Design review of the part built by this model. Coordinates are the model's own, in mm. A direction names the side the tool comes from. Give positions to 0.01 mm unless a question says otherwise; leave off trailing zeros. Write each loop counter-clockwise with the first axis right and the second up, starting at its lowest first coordinate (ties: lowest second). Pieces come first, ordered by that corner, then holes.
```python
from build123d import *

# Parameters (mm, degrees)
F0_W     = 30
F0_H     = 100
F1_DEPTH = 1.93
F3_D     = 10
F4_DEPTH = 1.93


# Not quite as in the source:
# - a feature names something its author has since deleted; it is built from what else it names


with BuildPart() as f1:
    # F0 (on Top) → F1 (new body)
    with BuildSketch(Plane.XY):
        with Locations((8.4595183283, 3.6650180817)):
            Rectangle(F0_W, F0_H)
    extrude(amount=F1_DEPTH)

    # F3 (through all)
    with Locations(Plane.XY.offset(1.93)):
        with Locations((8.4595183283, -36.3349819183)):
            Hole(F3_D / 2)

    # F2 (on face) → F4 (cut)
    with BuildSketch(Plane.XY.offset(1.93)):
        with BuildLine():
            Line((0.4595183283, 53.6650180817), (0.4595183283, 49.6650180817))
            ThreePointArc((0.4595183283, 49.6650180817), (8.4595183283, 41.6650180817), (16.4595183283, 49.6650180817))
            Line((16.4595183283, 49.6650180817), (16.4595183283, 53.6650180817))
            Line((16.4595183283, 53.6650180817), (0.4595183283, 53.6650180817))
        make_face()
    extrude(amount=-F4_DEPTH, mode=Mode.SUBTRACT)


solid = f1.part
```
(1) Clearance check with flat-ended pins moving along their axes: P1, Ø1, axis at x = 14.5, y = 40.5, coming from the -Z side; P2, Ø9, axis at x = 8.46, y = -36.33, coming from the +Z side (3 decimals). State where each tip first meets the part, or that it passes through.
Resolved:
P1: stops at z = 0
P2: passes through
(2) Mouldability with a two-part tool opening along X and no side actions: class faces 3 (the face through (0.46, 52, 1)), 4 (the face through (-6.54, 3, 1)), 5 (the face through (8, -46.335, 1)) as pulls with the +X half, pulls with the -X half, needs draft (parallel to the pull), parting line crosses it, or undercut.
Resolved:
face 3: undercut
face 4: pulls with the -X half
face 5: needs draft
(3) Tool access review of faces 1 (the face through (16.46, 52, 1)), 2 (the face through (8, 4, 1.93)): name each direction out of +Z, -Z, +X, -X, +Y, -Y from which nothing blocks a thin tool from reaching the whole face with its end or side.
Resolved:
face 1: +Z, -Z, +Y
face 2: +Z, +X, -X, +Y, -Y
(4) Consider section A-A, the plane y = 46. Give the boundary of the cut face in (x, z), then the cut area to 3 significant figures.
Resolved:
outline: (-6.54, 0) - (1.35, 0) - (1.35, 1.93) - (-6.54, 1.93) - close; (15.57, 0) - (23.46, 0) - (23.46, 1.93) - (15.57, 1.93) - close
area: 30.5 mm2
(5) To check wall thickness, follow L1, parallel to Y at x = 8.75, z = 1.25; L2, parallel to Y at x = 7, z = 1.4; L3, parallel to Y at x = 15, z = 0.8. State the ranges of each line that lie inside material, in increasing order.
Resolved:
L1: y = -46.33 to -41.33, -31.34 to 41.67
L2: y = -46.33 to -41.12, -31.55 to 41.8
L3: y = -46.33 to 45.06
(6) Consider section C-C, the plane y = -34. Give the boundary of the cut face in (x, z).
Resolved:
outline: (-6.54, 0) - (4.04, 0) - (4.04, 1.93) - (-6.54, 1.93) - close; (12.88, 0) - (23.46, 0) - (23.46, 1.93) - (12.88, 1.93) - close
(7) Consider section B-B, the plane z = 0.95. Give the boundary of the cut face in (x, y), then the cut area to 3 significant figures.
Resolved:
outline: (-6.54, -46.33) - (23.46, -46.33) - (23.46, 53.67) - (16.46, 53.67) - (16.46, 49.67) arc R8 cw to (0.46, 49.67) - (0.46, 53.67) - (-6.54, 53.67) - close; hole circle Ø10 at (8.46, -36.33)
area: 2,760 mm2
